from build123d import *

# Parameters (mm, degrees)
SKETCH1_W           = 15.24
SKETCH1_H           = 19.05
SKETCH1_R           = 3.302
BOSS_EXTRUDE1_DEPTH = 12.7762
CUT_EXTRUDE1_START  = -9.6012
SKETCH2_R           = 4.826
SKETCH2_R_2         = 3.302
CUT_EXTRUDE1_DEPTH  = 9.6012
SKETCH4_R           = 6.477
CUT_EXTRUDE4_DEPTH  = 1.5875
SKETCH5_R           = 0.635
CUT_EXTRUDE5_DEPTH  = 2.54


with BuildPart() as part:
    # Sketch1 → Boss-Extrude1 (new body)
    with BuildSketch(Plane.XY):
        with Locations((7.62, 9.525)):
            Rectangle(SKETCH1_W, SKETCH1_H)
        with Locations((7.62, 7.62)):
            Circle(SKETCH1_R, mode=Mode.SUBTRACT)
    extrude(amount=BOSS_EXTRUDE1_DEPTH)

    # Sketch2 → Cut-Extrude1 (cut)
    with BuildSketch(Plane.XY.offset(12.7762).offset(CUT_EXTRUDE1_START)):
        with Locations((7.62, 7.62)):
            Circle(SKETCH2_R)
        with Locations(Location((7.62, 7.62, 0), (0, 0, 180))):
            Circle(SKETCH2_R_2, mode=Mode.SUBTRACT)
    extrude(amount=CUT_EXTRUDE1_DEPTH, mode=Mode.SUBTRACT)

    # Sketch4 → Cut-Extrude4 (cut)
    with BuildSketch(Plane.XY.offset(12.7762)):
        with Locations((7.62, 7.62)):
            Circle(SKETCH4_R)
    extrude(amount=-CUT_EXTRUDE4_DEPTH, mode=Mode.SUBTRACT)

    # Sketch5 → Cut-Extrude5 (cut)
    with BuildSketch(Plane(origin=(0, 19.05, 0), x_dir=(1, 0, 0), z_dir=(0, 1, 0))):
        with Locations(Location((7.62, -8.517466667, 0), (0, 0, 270))):
            Circle(SKETCH5_R)
        with Locations(Location((7.62, -4.258733333, 0), (0, 0, 270))):
            Circle(SKETCH5_R)
    extrude(amount=-CUT_EXTRUDE5_DEPTH, mode=Mode.SUBTRACT)


solid = part.part
Geometry: final body of the model. Coordinates: model frame, mm. A direction names the side the tool comes from. Give positions to 0.01 mm unless a question says otherwise; leave off trailing zeros. Write each loop counter-clockwise with the first axis right and the second up, starting at its lowest first coordinate (ties: lowest second). Pieces come first, ordered by that corner, then holes. Notation, with made-up numbers: (17.25, 32.5) -> (31.25, 32.5) arc R14 cw to (31.25, 46.5) -> close; hole circle Ø3 at (-39, 65.5). An arc over 180 degrees is marked (long way). Answer as a JSON object with one key per item and string values.
1. Cut plane B-B on z = 6.5. Output: boundary loops of the cut face in (x, y).
Ans:
{"outline": "(0, 0) -> (15.24, 0) -> (15.24, 19.05) -> (0, 19.05) -> close; hole circle Ø9.65 at (7.62, 7.62)"}
2. Cut plane A-A on x = 7.62. Output: boundary loops of the cut face in (y, z) (3 decimals).
Ans:
{"outline": "(0, 0) -> (4.318, 0) -> (4.318, 3.175) -> (2.794, 3.175) -> (2.794, 11.189) -> (1.143, 11.189) -> (1.143, 12.776) -> (0, 12.776) -> close; (10.922, 0) -> (19.05, 0) -> (19.05, 3.624) -> (16.51, 3.624) -> (16.51, 4.894) -> (19.05, 4.894) -> (19.05, 7.882) -> (16.51, 7.882) -> (16.51, 9.152) -> (19.05, 9.152) -> (19.05, 12.776) -> (14.097, 12.776) -> (14.097, 11.189) -> (12.446, 11.189) -> (12.446, 3.175) -> (10.922, 3.175) -> close"}
3. Mould query, pull axis Y, two halves, no side actions, for faces 1 (the cylindrical face through (2.8, 7.83, 7.13)), 2 (the flat face through (0, 9, 6)), 3 (the flat face through (8, 19.05, 6)), 4 (the flat face through (8, 0, 6)). Classes: pulls with the +Y half, pulls with the -Y half, needs draft (parallel to the pull), parting line crosses it, or undercut.
Ans:
{"face 1": "undercut", "face 2": "needs draft", "face 3": "pulls with the +Y half", "face 4": "pulls with the -Y half"}
4. Access query for faces 5 (the flat face through (7.6, 16.51, 8.5)), 6 (the cylindrical face through (10.77, 8.61, 1.57)), 7 (the flat face through (3, 5, 11.189)). Directions: +Z, -Z, +X, -X, +Y, -Y. A direction counts if a zero-diameter tool reaches every point of the face in a straight line with its end or side. Return the directions, or none.
Ans:
{"face 5": "+Y", "face 6": "+Z, -Z", "face 7": "+Z"}
5. Contact query for flat-ended pins moving along their axis: pin 1 (1.5 mm diameter, centred on x = 13.5, z = 11, fed in from -Y); pin 2 (3 mm diameter, centred on x = 7, y = 9.5, fed in from +Z) (3 decimals); pin 3 (4 mm diameter, centred on x = 7.62, y = 7.62, fed in from -Z). Output: stop coordinate, or through.
Ans:
{"pin 1": "stops at y = 0", "pin 2": "stops at z = 3.175", "pin 3": "passes through"}
6. Ray query, probe 1 along Z at (x, y) = (7.75, 17); probe 2 along Y at (x, z) = (7.62, 8); probe 3 along X at (y, z) = (18, 8.5). Return the intervals inside material, ascending. Write a range as from..to.
Ans:
{"probe 1": "z = 0..3.64, 4.88..7.9, 9.14..12.78", "probe 2": "y = 0..2.79, 12.45..16.51", "probe 3": "x = 0..6.99, 8.25..15.24"}
7. Cut plane C-C on y = 7.62. Output: boundary loops of the cut face in (x, z) (3 decimals).
Ans:
{"outline": "(0, 0) -> (4.318, 0) -> (4.318, 3.175) -> (2.794, 3.175) -> (2.794, 11.189) -> (1.143, 11.189) -> (1.143, 12.776) -> (0, 12.776) -> close; (10.922, 0) -> (15.24, 0) -> (15.24, 12.776) -> (14.097, 12.776) -> (14.097, 11.189) -> (12.446, 11.189) -> (12.446, 3.175) -> (10.922, 3.175) -> close"}
8. Cut plane D-D on x = 13.5. Output: boundary loops of the cut face in (y, z), and give its area (3 significant figures).
Ans:
{"outline": "(0, 0) -> (19.05, 0) -> (19.05, 12.78) -> (10.34, 12.78) -> (10.34, 11.19) -> (4.9, 11.19) -> (4.9, 12.78) -> (0, 12.78) -> close", "area": "235 mm^2"}
